Verification items for the finished model (mm, model axes). Face numbers are marked on the shaded views. A direction names the side the tool comes from. Give positions to 0.01 mm unless a question says otherwise; leave off trailing zeros. Loops run counter-clockwise (first coordinate to the right, second up) from the corner with the lowest first, then second, coordinate; pieces in that order, holes last. Notation, with made-up numbers: M 45,45 L 69,45 A16 cw 69,67 Z; hole C -8.75,21.5 d2. An arc over 180 degrees is marked long. Put each result on its own line as item: value. Start each with the question number.
from build123d import *

# Parameters (mm, degrees)
F0_W     = 13.4
F0_H     = 26.3
F1_DEPTH = 5.8
F0_W_2   = 3.2
F0_H_2   = 23.3
F2_DEPTH = 2
F0_W_3   = 7.2
F3_DEPTH = 4.7


with BuildPart() as f1:
    # F0 (on Top) → F1 (new body)
    with BuildSketch(Plane.XY):
        with Locations((-14.642743, -19.200002)):
            Rectangle(F0_W, F0_H)
        Polygon((-19.842743, -30.850002), (-19.842743, -7.550002), (-16.642743, -7.550002), (-9.442743, -7.550002), (-9.442743, -30.850002), (-16.642743, -30.850002), align=None, mode=Mode.SUBTRACT)
    extrude(amount=-F1_DEPTH)

    # F0 (on Top) → F2 (join)
    with BuildSketch(Plane.XY):
        with Locations((-18.242743, -19.200002)):
            Rectangle(F0_W_2, F0_H_2)
    extrude(amount=-F2_DEPTH)

    # F0 (on Top) → F3 (join)
    with BuildSketch(Plane.XY):
        with Locations((-13.042743, -19.200002)):
            Rectangle(F0_W_3, F0_H_2)
    extrude(amount=-F3_DEPTH)


solid = f1.part
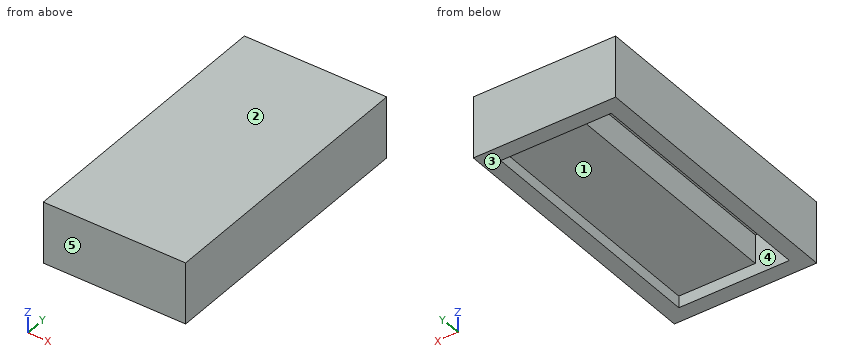
Q1. Set-up check for the marked faces 1 and 2: record each of +Z, -Z, +X, -X, +Y, -Y from which the full face is reachable in a straight line by a thin tool's end or side.
Q2. Scan lines: L1, parallel to Y at x = -18, z = -2.1; L2, parallel to X at y = -18.5, z = -2.4; L3, parallel to X at y = -27.5, z = -5. Record each from-to range of solid material in increasing order.
Q3. Cross-section at D-D, the plane x = -15.5. Record the boundary of the cut face in (y, z), then the cut area to 3 significant figures.
Q4. Release check for a two-part mould opening along Y. For the marked faces 3, 4 and 5 record: pulls with the +Y half, pulls with the -Y half, needs draft (parallel to the pull), parting line crosses it, or undercut.
Q5. Cross-section at B-B, the plane x = -19.5. Record the boundary of the cut face in (y, z), then the cut area to 3 significant figures.
Q6. Cross-section at C-C, the plane y = -25.5. Record the boundary of the cut face in (x, z), then the cut area to 3 significant figures.
Q7. Cross-section at A-A, the plane z = -4.2. Record the boundary of the cut face in (x, y).
Q8. Go/stop test with flat-tipped pins: pin 1 (4 mm diameter, centred on x = -10.5, y = -20.5, fed in from +Z); pin 2 (2.5 mm diameter, centred on x = -18.5, y = -21.5, fed in from -Z); pin 3 (2 mm diameter, centred on x = -16, y = -18, fed in from -Z). Record where each tip stops, or that it passes through.
Ans:
1. face 1: -Z
1. face 2: +Z, +X, -X, +Y, -Y
2. L1: y = -32.35 to -30.85, -7.55 to -6.05
2. L2: x = -21.34 to -19.84, -16.64 to -7.94
2. L3: x = -21.34 to -19.84, -9.44 to -7.94
3. outline: M -32.35,-5.8 L -30.85,-5.8 L -30.85,-4.7 L -7.55,-4.7 L -7.55,-5.8 L -6.05,-5.8 L -6.05,0 L -32.35,0 Z
3. area: 127 mm^2
4. face 3: needs draft
4. face 4: undercut
4. face 5: pulls with the -Y half
5. outline: M -32.35,-5.8 L -30.85,-5.8 L -30.85,-2 L -7.55,-2 L -7.55,-5.8 L -6.05,-5.8 L -6.05,0 L -32.35,0 Z
5. area: 64.0 mm^2
6. outline: M -21.34,-5.8 L -19.84,-5.8 L -19.84,-2 L -16.64,-2 L -16.64,-4.7 L -9.44,-4.7 L -9.44,-5.8 L -7.94,-5.8 L -7.94,0 L -21.34,0 Z
6. area: 57.6 mm^2
7. outline: M -21.34,-32.35 L -7.94,-32.35 L -7.94,-6.05 L -21.34,-6.05 Z; hole M -19.84,-30.85 L -16.64,-30.85 L -16.64,-7.55 L -19.84,-7.55 Z
8. pin 1: stops at z = 0
8. pin 2: stops at z = -2
8. pin 3: stops at z = -4.7
